The model under review builds one solid part; all positions refer to its coordinate system, in mm. A direction names the side the tool comes from. Give positions to 0.01 mm unless a question says otherwise; leave off trailing zeros. Loops run counter-clockwise (first coordinate to the right, second up) from the corner with the lowest first, then second, coordinate; pieces in that order, holes last. Notation, with made-up numbers: M 86,30 L 115,30 A26 ccw 115,45 Z; hole C -29.75,38.5 d4. An arc over 180 degrees is marked long. Return JSON: item names as keys, results as strings. Group by question number.
```python
from build123d import *

# Parameters (mm, degrees)
SKETCH_1_W          = 20
SKETCH_1_H          = 18
EXTRUDE_1_DEPTH     = 4
SKETCH_2_W          = 3
SKETCH_2_H          = 18
EXTRUDE_2_DEPTH     = 10
CUT_EXTRUDE_1_DEPTH = 28.856776554
SKETCH_6_R          = 2.5
CUT_EXTRUDE_2_DEPTH = 28.856776554
FILLET_1_R          = 3
SKETCH_9_W          = 4
SKETCH_9_H          = 18
CUT_EXTRUDE_4_DEPTH = 29.705400189
SKETCH_10_W         = 4
SKETCH_10_H         = 18
CUT_EXTRUDE_5_DEPTH = 29.705400189
SKETCH_11_R         = 1.5
CUT_EXTRUDE_6_DEPTH = 27.076809621
SKETCH_12_R         = 2.75
CUT_EXTRUDE_7_DEPTH = 2


with BuildPart() as part:
    # 草图1 → 凸台-拉伸1 (new body)
    with BuildSketch(Plane.XY):
        with Locations((10, 9)):
            Rectangle(SKETCH_1_W, SKETCH_1_H)
    extrude(amount=EXTRUDE_1_DEPTH)

    # 草图2 → 凸台-拉伸2 (add)
    with BuildSketch(Plane.XY.offset(4)):
        with Locations((14.5, 9)):
            Rectangle(SKETCH_2_W, SKETCH_2_H)
        with Locations((5.5, 9)):
            Rectangle(SKETCH_2_W, SKETCH_2_H)
    extrude(amount=EXTRUDE_2_DEPTH)

    # 草图3 → 切除-拉伸1 (cut, through all)
    with BuildSketch(Plane.ZY.offset(-4)):
        Polygon((4, 18), (14, 13), (14, 19.313508938), align=None)
        Polygon((4, 0), (14, 5), (15.372444732, -0.863940538), align=None)
    extrude(amount=-CUT_EXTRUDE_1_DEPTH, mode=Mode.SUBTRACT)

    # 草图6 → 切除-拉伸2 (cut, through all)
    with BuildSketch(Plane(origin=(16, 0, 0), x_dir=(0, 0, -1), z_dir=(1, 0, 0))):
        with Locations(Location((-9, 9, 0), (0, 0, 90))):
            Circle(SKETCH_6_R)
    extrude(amount=-CUT_EXTRUDE_2_DEPTH, mode=Mode.SUBTRACT)

    # 圆角1
    fillet_1_edges = [part.edges().sort_by_distance(p)[0] for p in [
        (5.5, 13, 14),
        (14.5, 13, 14),
        (5.5, 5, 14),
        (14.5, 5, 14),
    ]]
    fillet(fillet_1_edges, radius=FILLET_1_R)

    # 草图9 → 切除-拉伸4 (cut, through all)
    with BuildSketch(Plane.XY.offset(4)):
        with Locations((2, 9)):
            Rectangle(SKETCH_9_W, SKETCH_9_H)
    extrude(amount=-CUT_EXTRUDE_4_DEPTH, mode=Mode.SUBTRACT)

    # 草图10 → 切除-拉伸5 (cut, through all)
    with BuildSketch(Plane.XY.offset(4)):
        with Locations((18, 9)):
            Rectangle(SKETCH_10_W, SKETCH_10_H)
    extrude(amount=-CUT_EXTRUDE_5_DEPTH, mode=Mode.SUBTRACT)

    # 草图11 → 切除-拉伸6 (cut, through all)
    with BuildSketch(Plane.XY.offset(4)):
        with Locations((10, 14)):
            Circle(SKETCH_11_R)
        with Locations((10, 4)):
            Circle(SKETCH_11_R)
    extrude(amount=-CUT_EXTRUDE_6_DEPTH, mode=Mode.SUBTRACT)

    # 草图12 → 切除-拉伸7 (cut)
    with BuildSketch(Plane.XY.offset(4)):
        with Locations((10, 14)):
            Circle(SKETCH_12_R)
        with Locations((10, 4)):
            Circle(SKETCH_12_R)
    extrude(amount=-CUT_EXTRUDE_7_DEPTH, mode=Mode.SUBTRACT)


solid = part.part
```
(1) Mouldability with a two-part tool opening along Y and no side actions: class faces 1 (the cylindrical face through (5.52, 8.46, 6.56)), 2 (the cylindrical face through (14.52, 12.74, 13.54)), 3 (the flat face through (4, 9, 6)), 4 (the flat face through (11.2, 12.8, 2)) as released by +Y, released by -Y, zero draft, split by the parting line, or undercut.
(2) Add section A-A (z = 9). Write out the cut boundary in (x, y).
(3) Add section B-B (y = 9). Write out the cut boundary in (x, z).
(4) For pin 1 (5 mm diameter, centred on x = 5.5, y = 12.5, fed in from -Z); pin 2 (1.8 mm diameter, centred on x = 10, y = 4, fed in from +Z); pin 3 (6 mm diameter, centred on x = 7, z = 10.5, fed in from +Y); pin 4 (6 mm diameter, centred on x = 9, y = 4.5, fed in from +Z), all flat-tipped, find the tip position at first contact; note any pin that passes through.
(5) For faces 5 (the flat face through (5, 9, 14)), 6 (the flat face through (11.2, 2.8, 2)), 7 (the flat face through (7, 11, 7)), list the 3-axis set-ups (+Z, -Z, +X, -X, +Y, -Y) from which the entire face can be reached by the end or side of a thin tool; tool diameter is ignored.
(6) Add section D-D (z = 4.5). Write out the cut boundary in (x, y), and give its area (3 significant figures).
(7) Add section C-C (x = 10). Write out the cut boundary in (y, z).
(8) For probe 1 along Y at (x, z) = (10, 3.1); probe 2 along Y at (x, z) = (10, 1.25); probe 3 along Z at (x, y) = (13.9, 9), list the stretches that pass through material, from the lowest coordinate up.
Verdict:
{
 "1": {"face 1": "undercut", "face 2": "released by +Y", "face 3": "zero draft", "face 4": "undercut"},
 "2": {"outline": "M 4,2.5 L 7,2.5 L 7,6.5 L 4,6.5 Z; M 4,11.5 L 7,11.5 L 7,15.5 L 4,15.5 Z; M 13,2.5 L 16,2.5 L 16,6.5 L 13,6.5 Z; M 13,11.5 L 16,11.5 L 16,15.5 L 13,15.5 Z"},
 "3": {"outline": "M 4,0 L 16,0 L 16,6.5 L 13,6.5 L 13,4 L 7,4 L 7,6.5 L 4,6.5 Z; M 4,11.5 L 7,11.5 L 7,14 L 4,14 Z; M 13,11.5 L 16,11.5 L 16,14 L 13,14 Z"},
 "4": {"pin 1": "stops at z = 0", "pin 2": "passes through", "pin 3": "stops at y = 16.25", "pin 4": "stops at z = 14"},
 "5": {"face 5": "+Z, +X, -X, +Y, -Y", "face 6": "+Z", "face 7": "+Z, +Y, -Y"},
 "6": {"outline": "M 4,0.25 L 7,0.25 L 7,17.75 L 4,17.75 Z; M 13,0.25 L 16,0.25 L 16,17.75 L 13,17.75 Z", "area": "105 mm²"},
 "7": {"outline": "M 0,0 L 2.5,0 L 2.5,2 L 1.25,2 L 1.25,4 L 0,4 Z; M 5.5,0 L 12.5,0 L 12.5,2 L 11.25,2 L 11.25,4 L 6.75,4 L 6.75,2 L 5.5,2 Z; M 15.5,0 L 18,0 L 18,4 L 16.75,4 L 16.75,2 L 15.5,2 Z"},
 "8": {"probe 1": "y = 0 to 1.25, 6.75 to 11.25, 16.75 to 18", "probe 2": "y = 0 to 2.5, 5.5 to 12.5, 15.5 to 18", "probe 3": "z = 0 to 6.5, 11.5 to 14"}
}
